Geometry: final body of the model. Coordinates: model frame, mm. Face numbers are marked on the shaded views. A direction names the side the tool comes from. Coordinates: 2 decimals unless noted, no trailing zeros. Order: outer loops, then holes, each group sorted by start corner. A loop starts at its lowest first (then second) coordinate and runs counter-clockwise, first axis right, second up. Notation, with made-up numbers: M -23.5,64 L 27.5,64 A32 cw 27.5,99 Z; hole C -3.5,38 d7. An arc over 180 degrees is marked long. Use CSV: the item, a comma, the result in double quotes. Start each with the question number.
Q1. Section query D-D, the plane y = 7.75. Output: boundary loops of the cut face in (x, z).
Q2. Ray query, probe 1 along Z at (x, y) = (45, 11.1); probe 2 along X at (y, z) = (11.4, -25); probe 3 along X at (y, z) = (10.5, -26). Return the intervals inside material, ascending.
Q3. Section query C-C, the plane x = 3. Output: boundary loops of the cut face in (y, z), and give its area (3 significant figures).
Q4. First-contact query: P1, Ø2.5, axis at x = 22, z = -27, coming from the -Y side; P2, Ø5, axis at x = 22, y = 6.5, coming from the +Z side; P3, Ø2.5, axis at x = -45, z = 25, coming from the -Y side. Flat tips, straight axial feed; report the tip coordinate or a pass-through.
Q5. Section query A-A, the plane x = 45. Output: boundary loops of the cut face in (y, z).
Q6. Section query B-B, the plane z = 25. Output: boundary loops of the cut face in (x, y).
Q7. Access query for the marked faces 1 and 2. Directions: +Z, -Z, +X, -X, +Y, -Y. A direction counts if a zero-diameter tool reaches every point of the face in a straight line with its end or side. Return the directions, or none.
from build123d import *

# Parameters (mm, degrees)
SKETCH1_W           = 101.6
SKETCH1_H           = 60.325
BOSS_EXTRUDE1_DEPTH = 12
SKETCH2_W           = 9.1625
SKETCH2_H           = 10
CUT_EXTRUDE1_DEPTH  = 102.6
SKETCH3_R           = 1.5
CUT_EXTRUDE2_DEPTH  = 13


with BuildPart() as part:
    # Sketch1 → Boss-Extrude1 (new body)
    with BuildSketch(Plane(origin=(0, 0, 0), x_dir=(1, 0, 0), z_dir=(0, 1, 0))):
        Rectangle(SKETCH1_W, SKETCH1_H)
    extrude(amount=BOSS_EXTRUDE1_DEPTH)

    # Sketch2 → Cut-Extrude1 (cut, through all)
    with BuildSketch(Plane(origin=(50.8, 0, 0), x_dir=(0, 0, -1), z_dir=(1, 0, 0))):
        with Locations((-25.58125, 5)):
            Rectangle(SKETCH2_W, SKETCH2_H)
        with Locations((25.58125, 5)):
            Rectangle(SKETCH2_W, SKETCH2_H)
    extrude(amount=-CUT_EXTRUDE1_DEPTH, mode=Mode.SUBTRACT)

    # Sketch3 → Cut-Extrude2 (cut, through all)
    with BuildSketch(Plane(origin=(0, 12, 0), x_dir=(1, 0, 0), z_dir=(0, 1, 0))):
        with Locations((-45, 25)):
            Circle(SKETCH3_R)
        with Locations((-45, -25)):
            Circle(SKETCH3_R)
        with Locations((45, -25)):
            Circle(SKETCH3_R)
        with Locations((45, 25)):
            Circle(SKETCH3_R)
    extrude(amount=-CUT_EXTRUDE2_DEPTH, mode=Mode.SUBTRACT)


solid = part.part
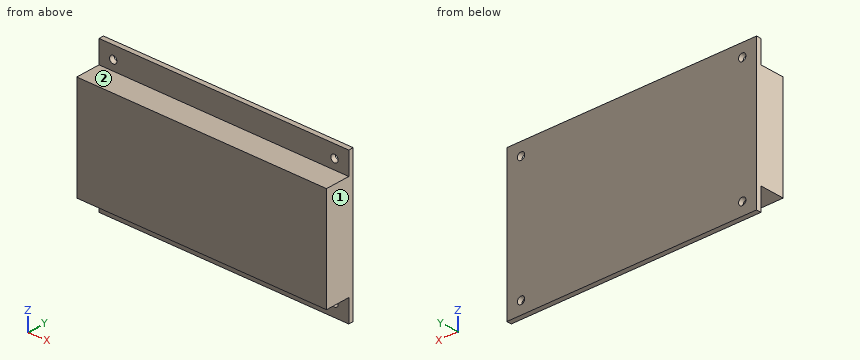
Responses:
1,outline,"M -50.8,-21 L 50.8,-21 L 50.8,21 L -50.8,21 Z"
2,probe 1,"z = -30.16 to -26.5, -23.5 to 23.5, 26.5 to 30.16"
2,probe 2,"x = -50.8 to -46.5, -43.5 to 43.5, 46.5 to 50.8"
2,probe 3,"x = -50.8 to -46.12, -43.88 to 43.88, 46.12 to 50.8"
3,outline,"M 0,-21 L 10,-21 L 10,-30.16 L 12,-30.16 L 12,30.16 L 10,30.16 L 10,21 L 0,21 Z"
3,area,"541 mm²"
4,P1,"stops at y = 10"
4,P2,"stops at z = 21"
4,P3,"passes through"
5,outline,"M 0,-21 L 10,-21 L 10,-23.5 L 12,-23.5 L 12,23.5 L 10,23.5 L 10,21 L 0,21 Z; M 10,-30.16 L 12,-30.16 L 12,-26.5 L 10,-26.5 Z; M 10,26.5 L 12,26.5 L 12,30.16 L 10,30.16 Z"
6,outline,"M -50.8,10 L -46.5,10 L -46.5,12 L -50.8,12 Z; M -43.5,10 L 43.5,10 L 43.5,12 L -43.5,12 Z; M 46.5,10 L 50.8,10 L 50.8,12 L 46.5,12 Z"
7,face 1,"+Z, -Z, +X, +Y, -Y"
7,face 2,"+Z, +X, -X, -Y"
